Geometry: final body of the model. Coordinates: model frame, mm. Face numbers are marked on the shaded views. Give positions to 0.01 mm unless a question says otherwise; leave off trailing zeros. Write each loop counter-clockwise with the first axis right and the second up, starting at its lowest first coordinate (ties: lowest second). Pieces come first, ordered by that corner, then holes.
Q1. Cut plane C-C on x = 10.5. Return the cut outline in (y, z).
Q2. Pin query (flat end, axial travel): pin 1 (0.9 mm diameter, centred on y = 140.5, z = -1, fed in from -X); pin 2 (1.5 mm diameter, centred on x = 15, z = -2, fed in from +Y); pin 3 (2.5 mm diameter, centred on y = 144, z = -2, fed in from +X). Return the tip coordinate at first contact, or that it passes through.
Q3. Cut plane B-B on y = 98. Return the cut outline in (x, z), plus the area to 4 significant figures.
Q4. Line query: L1, parallel to X at y = 40.5, z = 34; L2, parallel to Y at x = 21, z = 19.5; L3, parallel to Z at x = 2.5, y = 203. Output: solid intervals per line, ascending.
Q5. Draft query along X for the marked faces 1, 2, 3 and 4. Return one class per face: pulls with the +X half, pulls with the -X half, needs draft (parallel to the pull), parting line crosses it, or undercut.
Q6. Cut plane A-A on z = 10. Return the cut outline in (x, y).
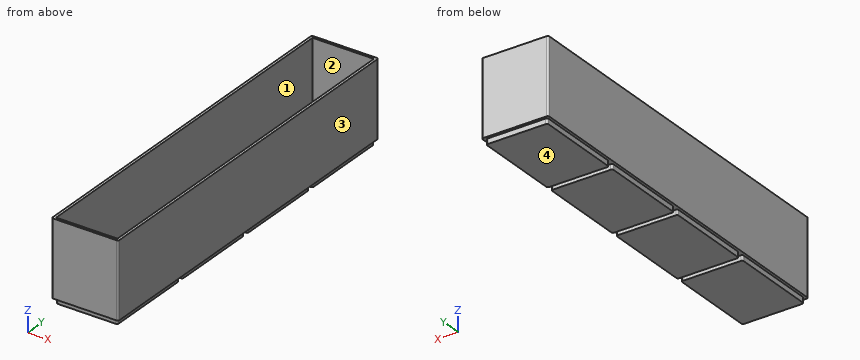
```python
from build123d import *

# Parameters (mm, degrees)
F0_W     = 35
F0_H     = 50
F1_DEPTH = 3
F0_H_2   = 1.5
F2_DEPTH = 1.5
F3_DEPTH = 43
F4_R     = 1


with BuildPart() as f1:
    # F0 (on Top) → F1 (new body)
    with BuildSketch(Plane.XY):
        with Locations((19, 185.5)):
            Rectangle(F0_W, F0_H)
        with Locations((19, 132.5)):
            Rectangle(F0_W, F0_H)
        with Locations((19, 79.5)):
            Rectangle(F0_W, F0_H)
        with Locations((19, 26.5)):
            Rectangle(F0_W, F0_H)
    extrude(amount=-F1_DEPTH)

    # F0 (on Top) → F2 (join)
    with BuildSketch(Plane.XY):
        with Locations((19, 185.5)):
            Rectangle(F0_W, F0_H)
        Polygon((0, 212), (0, 159), (1.5, 159), (1.5, 160.5), (1.5, 210.5), (36.5, 210.5), (36.5, 160.5), (36.5, 159), (38, 159), (38, 212), align=None)
        with Locations((19, 132.5)):
            Rectangle(F0_W, F0_H)
        Polygon((36.5, 106), (38, 106), (38, 159), (36.5, 159), (36.5, 157.5), (36.5, 107.5), align=None)
        with Locations((19, 158.25)):
            Rectangle(F0_W, F0_H_2)
        with Locations((19, 159.75)):
            Rectangle(F0_W, F0_H_2)
        Polygon((0, 159), (0, 106), (1.5, 106), (1.5, 107.5), (1.5, 157.5), (1.5, 159), align=None)
        with Locations((19, 105.25)):
            Rectangle(F0_W, F0_H_2)
        with Locations((19, 106.75)):
            Rectangle(F0_W, F0_H_2)
        Polygon((36.5, 53), (38, 53), (38, 106), (36.5, 106), (36.5, 104.5), (36.5, 54.5), align=None)
        with Locations((19, 79.5)):
            Rectangle(F0_W, F0_H)
        Polygon((0, 106), (0, 53), (1.5, 53), (1.5, 54.5), (1.5, 104.5), (1.5, 106), align=None)
        Polygon((0, 53), (0, 0), (38, 0), (38, 53), (36.5, 53), (36.5, 51.5), (36.5, 1.5), (1.5, 1.5), (1.5, 51.5), (1.5, 53), align=None)
        with Locations((19, 26.5)):
            Rectangle(F0_W, F0_H)
        with Locations((19, 52.25)):
            Rectangle(F0_W, F0_H_2)
        with Locations((19, 53.75)):
            Rectangle(F0_W, F0_H_2)
    extrude(amount=F2_DEPTH)

    # F0 (on Top) → F3 (join)
    with BuildSketch(Plane.XY):
        Polygon((0, 53), (0, 0), (38, 0), (38, 53), (36.5, 53), (36.5, 51.5), (36.5, 1.5), (1.5, 1.5), (1.5, 51.5), (1.5, 53), align=None)
        Polygon((0, 106), (0, 53), (1.5, 53), (1.5, 54.5), (1.5, 104.5), (1.5, 106), align=None)
        Polygon((36.5, 53), (38, 53), (38, 106), (36.5, 106), (36.5, 104.5), (36.5, 54.5), align=None)
        Polygon((36.5, 106), (38, 106), (38, 159), (36.5, 159), (36.5, 157.5), (36.5, 107.5), align=None)
        Polygon((0, 159), (0, 106), (1.5, 106), (1.5, 107.5), (1.5, 157.5), (1.5, 159), align=None)
        Polygon((0, 212), (0, 159), (1.5, 159), (1.5, 160.5), (1.5, 210.5), (36.5, 210.5), (36.5, 160.5), (36.5, 159), (38, 159), (38, 212), align=None)
    extrude(amount=F3_DEPTH)

    # F4
    f4_edges = [f1.edges().sort_by_distance(p)[0] for p in [
        (38, 212, 21.5),
        (0, 212, 21.5),
        (1.5, 210.5, -1.5),
        (36.5, 210.5, -1.5),
        (1.5, 160.5, -1.5),
        (36.5, 160.5, -1.5),
        (36.5, 157.5, -1.5),
        (1.5, 157.5, -1.5),
        (1.5, 107.5, -1.5),
        (36.5, 107.5, -1.5),
        (36.5, 104.5, -1.5),
        (1.5, 104.5, -1.5),
        (1.5, 54.5, -1.5),
        (36.5, 54.5, -1.5),
        (36.5, 51.5, -1.5),
        (1.5, 51.5, -1.5),
        (1.5, 1.5, -1.5),
        (36.5, 1.5, -1.5),
        (38, 0, 21.5),
        (0, 0, 21.5),
    ]]
    fillet(f4_edges, radius=F4_R)


solid = f1.part
```
Data:
1. outline: (0, 0) - (1.5, 0) - (1.5, -3) - (51.5, -3) - (51.5, 0) - (54.5, 0) - (54.5, -3) - (104.5, -3) - (104.5, 0) - (107.5, 0) - (107.5, -3) - (157.5, -3) - (157.5, 0) - (160.5, 0) - (160.5, -3) - (210.5, -3) - (210.5, 0) - (212, 0) - (212, 43) - (210.5, 43) - (210.5, 1.5) - (1.5, 1.5) - (1.5, 43) - (0, 43) - close
2. pin 1: stops at x = 1.5
2. pin 2: stops at y = 210.5
2. pin 3: stops at x = 36.5
3. outline: (0, 0) - (1.5, 0) - (1.5, -3) - (36.5, -3) - (36.5, 0) - (38, 0) - (38, 43) - (36.5, 43) - (36.5, 1.5) - (1.5, 1.5) - (1.5, 43) - (0, 43) - close
3. area: 286.5 mm2
4. L1: x = 0 to 1.5, 36.5 to 38
4. L2: y = 0 to 1.5, 210.5 to 212
4. L3: z = -3 to 1.5
5. face 1: undercut
5. face 2: undercut
5. face 3: pulls with the +X half
5. face 4: needs draft
6. outline: (0, 1) arc R1 ccw to (1, 0) - (37, 0) arc R1 ccw to (38, 1) - (38, 211) arc R1 ccw to (37, 212) - (1, 212) arc R1 ccw to (0, 211) - close; hole (1.5, 1.5) - (36.5, 1.5) - (36.5, 210.5) - (1.5, 210.5) - close
